from build123d import *

# Parameters (mm, degrees)
F0_W     = 8.89
F0_H     = 19.05
F0_W_2   = 3.175
F0_H_2   = 7.62
F1_DEPTH = 12.7
F2_R     = 2.54
F3_R     = 2.413
F4_DEPTH = 25.4
F5_SIZE  = 7.62


with BuildPart() as f1:
    # F0 (on Top) → F1 (new body)
    with BuildSketch(Plane.XY):
        with Locations((-10.492269, 9.525)):
            Rectangle(F0_W, F0_H)
        Polygon((-6.047269, 0), (-14.937269, 0), (-14.937269, -6.35), (9.827731, -6.35), (9.827731, 0), (6.652731, 0), align=None)
        with Locations((8.240231, 3.81)):
            Rectangle(F0_W_2, F0_H_2)
    extrude(amount=F1_DEPTH)

    # F2
    f2_edges = [f1.edges().sort_by_distance(p)[0] for p in [
        (6.652731, 0, 6.35),
        (9.827731, -6.35, 6.35),
        (-14.937269, -6.35, 6.35),
    ]]
    fillet(f2_edges, radius=F2_R)

    # F3 (on face) → F4 (cut)
    with BuildSketch(Plane.YZ.offset(-6.047269)):
        with Locations((12.7, 6.35)):
            Circle(F3_R)
    extrude(amount=-F4_DEPTH, mode=Mode.SUBTRACT)

    # F5
    f5_edges = [f1.edges().sort_by_distance(p)[0] for p in [
        (-6.047269, 0, 6.35),
    ]]
    chamfer(f5_edges, length=F5_SIZE)


solid = f1.part
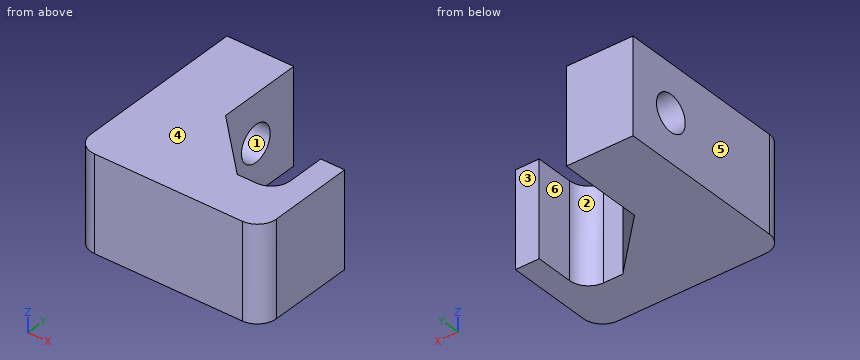
Build history of the part. All positions in model axes, mm. Face numbers are marked on the shaded views. A direction names the side the tool comes from. Round coordinates to 2 decimals unless told otherwise and drop trailing zeros. Loops run counter-clockwise (first coordinate to the right, second up) from the corner with the lowest first, then second, coordinate; pieces in that order, holes last. Notation, with made-up numbers: (5, -14) -> (45, -14) arc R17 cw to (45, 2) -> close; hole circle Ø9 at (33, 18.25). An arc over 180 degrees is marked (long way). Use CSV: the item, a comma, the result in double quotes. Start each with the question number.
Q1. Saw through at B-B on z = 6.35. Give the cut face in (x, y).
Q2. Mould opens along X. For the marked faces 4, 5 and 6 say: +X half, -X half, draft (parallel to the pull), parting line (faces both ways), or undercut.
Q3. Saw through at D-D on z = 11.5. Give the cut face in (x, y), and give its area (3 significant figures).
Q4. Saw through at A-A on y = 12.7. Give the cut face in (x, z).
Q5. Flat gauge pins, fed straight in: pin 1 Ø3 at (x, z) = (3.5, 5.5) entering from +Y; pin 2 Ø7.5 at (y, z) = (12.7, 6.35) entering from +X; pin 3 Ø1.6 at (x, z) = (7.5, 9) entering from +Y; pin 4 Ø8 at (x, y) = (5.5, 15) entering from -Z. Where does each tip first touch, or does it go through?
Q6. Which spindle directions (+Z, -Z, +X, -X, +Y, -Y) get a long thin tool onto all of the face, cutting with end or side? Do the marked faces 1, 2 and 3. Say none if no direction does.
Q7. Drill centre lines: L1, parallel to Z at x = -8.75, y = 12.7; L2, parallel to X at y = 13.75, z = 4; L3, parallel to X at y = 4.25, z = 9.5. Where is each one in solid material? Low to high.
Q8. Saw through at C-C on x = -10.25. Give the cut face in (y, z), and give its area (3 significant figures).
Solutions:
1,outline,"(-14.94, -3.81) arc R2.54 ccw to (-12.4, -6.35) -> (7.29, -6.35) arc R2.54 ccw to (9.83, -3.81) -> (9.83, 7.62) -> (6.65, 7.62) -> (6.65, 2.54) arc R2.54 cw to (4.11, 0) -> (1.57, 0) -> (-6.05, 7.62) -> (-6.05, 10.29) -> (-14.94, 10.29) -> close; (-14.94, 15.11) -> (-6.05, 15.11) -> (-6.05, 19.05) -> (-14.94, 19.05) -> close"
2,face 4,"draft"
2,face 5,"-X half"
2,face 6,"undercut"
3,outline,"(-14.94, -3.81) arc R2.54 ccw to (-12.4, -6.35) -> (7.29, -6.35) arc R2.54 ccw to (9.83, -3.81) -> (9.83, 7.62) -> (6.65, 7.62) -> (6.65, 2.54) arc R2.54 cw to (4.11, 0) -> (1.57, 0) -> (-6.05, 7.62) -> (-6.05, 19.05) -> (-14.94, 19.05) -> close"
3,area,"378 mm^2"
4,outline,"(-14.94, 0) -> (-6.05, 0) -> (-6.05, 3.94) -> (-14.94, 3.94) -> close; (-14.94, 8.76) -> (-6.05, 8.76) -> (-6.05, 12.7) -> (-14.94, 12.7) -> close"
5,pin 1,"stops at y = 0.16"
5,pin 2,"stops at x = -6.05"
5,pin 3,"stops at y = 7.62"
5,pin 4,"passes through"
6,face 1,"+X, -X"
6,face 2,"+Z, -Z, +Y"
6,face 3,"+Z, -Z, +X, +Y"
7,L1,"z = 0 to 3.94, 8.76 to 12.7"
7,L2,"x = -14.94 to -6.05"
7,L3,"x = -14.94 to -2.68, 6.65 to 9.83"
8,outline,"(-6.35, 0) -> (19.05, 0) -> (19.05, 12.7) -> (-6.35, 12.7) -> close; hole circle Ø4.83 at (12.7, 6.35)"
8,area,"304 mm^2"
